Here's how the part is built. I have some questions about the finished solid (model axes, mm). A direction names the side the tool comes from. Round coordinates to 2 decimals unless told otherwise and drop trailing zeros. Order: outer loops, then holes, each group sorted by start corner. A loop starts at its lowest first (then second) coordinate and runs counter-clockwise, first axis right, second up. Notation, with made-up numbers: (73.25, 34.25) -> (97.25, 34.25) arc R16 cw to (97.25, 47.25) -> close; hole circle Ø4 at (47, 20.25). An arc over 180 degrees is marked (long way). Use a Markdown table: item, result. Add a question column.
(1) I want a section at B-B, the plane x = -14. Please give me the cut outline in (y, z).
(2) I want a section at C-C, the plane z = -1.5. Please give me the cut outline in (x, y).
(3) Thinking about a two-plate mould opening in X: for faces 5 (the face through (-2, 2, 5.124)), 6 (the face through (0.68, 5.48, -6.83)), 7 (the face through (-14.874, 5, -3)), which applies, pulls with the +X half, pulls with the -X half, needs draft (parallel to the pull), parting line crosses it, or undercut?
(4) On a 3-axis mill with a long thin cutter (end or side, diameter ignored), from which of +Z, -Z, +X, -X, +Y, -Y can I reach the whole of each face in a straight line? I mean faces 1 (the face through (-4.874, 5, -3)), 2 (the face through (0.6, 5.5, -1.9)), 3 (the face through (-10, 5, -0.876)), 4 (the face through (-10, 5, -5.876)). Say none if no direction works.
(5) I want a section at A-A, the plane y = 5.5. Please give me the cut outline in (x, z).
(6) I want a section at D-D, the plane x = 7. Please give me the cut outline in (y, z).
(7) I'm going to push flat-ended pins straight in: P1, Ø0.9, axis at x = -11.5, y = 5, coming from the +Z side; P2, Ø1.5, axis at x = -8, y = 5.5, coming from the -Z side; P3, Ø1, axis at y = 5, z = -4.5, coming from the -X side. Where does each tip first touch, or does it pass through?
(8) If I drill on probe 1 along Y at (x, z) = (16, 0.25); probe 2 along X at (y, z) = (4.25, -4.75); probe 3 along X at (y, z) = (5, -5.5), over which ranges is the centre line in solid material (lowest first)?
from build123d import *

# Parameters (mm, degrees)
SKETCH1_W           = 44
SKETCH1_H           = 18
BOSS_EXTRUDE1_DEPTH = 4
SKETCH2_W           = 10
SKETCH2_H           = 5
BOSS_EXTRUDE2_DEPTH = 3


with BuildPart() as part:
    # Sketch1 → Boss-Extrude1 (new body)
    with BuildSketch(Plane(origin=(0, 0, 0), x_dir=(1, 0, 0), z_dir=(0, 1, 0))):
        with Locations((-1.926267281, 3.875576037)):
            Rectangle(SKETCH1_W, SKETCH1_H)
    extrude(amount=BOSS_EXTRUDE1_DEPTH)

    # Sketch2 → Boss-Extrude2 (add)
    with BuildSketch(Plane(origin=(0, 4, 0), x_dir=(1, 0, 0), z_dir=(0, 1, 0))):
        with Locations((-9.873666519, 3.375576037)):
            Rectangle(SKETCH2_W, SKETCH2_H)
        Polygon((-1.825762218, 4.325323505), (3.123985251, -0.624423963), (8.073732719, 4.325323505), (3.123985251, 9.275070973), align=None)
    extrude(amount=BOSS_EXTRUDE2_DEPTH)


solid = part.part
Taken from the geometry:
| question | item | result |
|---|---|---|
| 1 | outline | (0, -12.88) -> (4, -12.88) -> (4, -5.88) -> (7, -5.88) -> (7, -0.88) -> (4, -0.88) -> (4, 5.12) -> (0, 5.12) -> close |
| 2 | outline | (-23.93, 0) -> (20.07, 0) -> (20.07, 4) -> (5.25, 4) -> (5.25, 7) -> (1, 7) -> (1, 4) -> (-4.87, 4) -> (-4.87, 7) -> (-14.87, 7) -> (-14.87, 4) -> (-23.93, 4) -> close |
| 3 | face 5 | needs draft |
| 3 | face 6 | undercut |
| 3 | face 7 | pulls with the -X half |
| 4 | face 1 | +Z, -Z, +Y |
| 4 | face 2 | +Z, +Y |
| 4 | face 3 | +Z, -X, +Y |
| 4 | face 4 | -Z, -X, +Y |
| 5 | outline | (-14.87, -5.88) -> (-4.87, -5.88) -> (-4.87, -0.88) -> (-14.87, -0.88) -> close; (-1.83, -4.33) -> (3.12, -9.28) -> (8.07, -4.33) -> (3.12, 0.62) -> close |
| 6 | outline | (0, -12.88) -> (4, -12.88) -> (4, -5.4) -> (7, -5.4) -> (7, -3.25) -> (4, -3.25) -> (4, 5.12) -> (0, 5.12) -> close |
| 7 | P1 | stops at z = -0.88 |
| 7 | P2 | stops at z = -5.88 |
| 7 | P3 | stops at x = -14.87 |
| 8 | probe 1 | y = 0 to 4 |
| 8 | probe 2 | x = -14.87 to -4.87, -1.4 to 7.65 |
| 8 | probe 3 | x = -14.87 to -4.87, -0.65 to 6.9 |
